Can you work these out from the drawing? Everything is in mm from the part's minimum corner. Give positions to 0.01 mm unless a question says otherwise; leave off trailing zeros. Write each loop counter-clockwise with the first axis right and the second up, starting at its lowest first coordinate (ties: lowest second). Pieces come first, ordered by that corner, then holes. Notation, with made-up numbers: M 11.5,15.25 L 19.5,15.25 A24 ccw 19.5,49.25 Z; hole C 36,25 d5. An arc over 180 degrees is marked long. One line per item, written item: value.
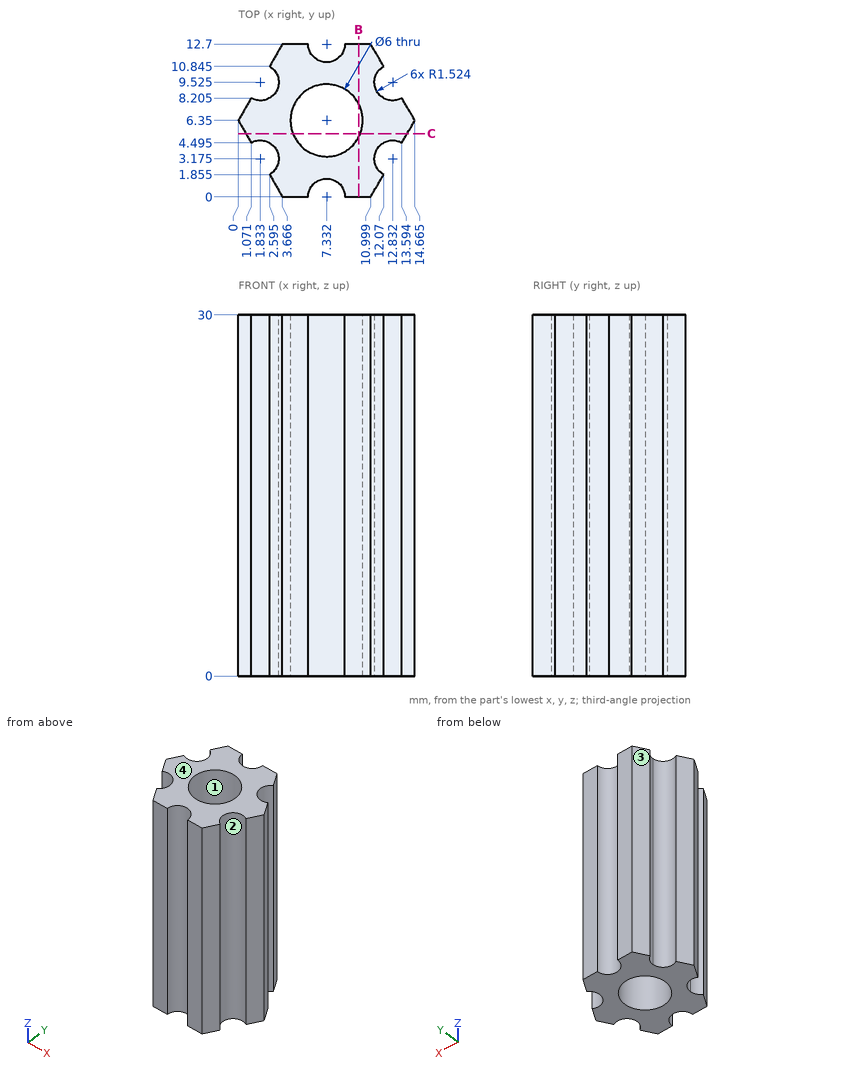
1) Please list where these lines run through material, in increasing order: L1, parallel to Y at x = 7.5, z = 19.75 (1 decimal); L2, parallel to Y at x = 5.5, z = 5.75 (1 decimal); L3, parallel to X at y = 8.5, z = 22.25 (1 decimal). Write a range as from..to.
Outcome:
L1: y = 1.5..3.4, 9.3..11.2
L2: y = 0..4, 8.7..12.7
L3: x = 3..5.2, 9.4..11.7
2) I'm going to push flat-ended pins straight in: pin 1 (1 mm diameter, centred on y = 11, z = 11, fed in from -X) (1 decimal); pin 2 (1 mm diameter, centred on y = 9, z = 9.5, fed in from -X). Where does each tip first touch, or does it pass through?
Outcome:
pin 1: stops at x = 2.6
pin 2: stops at x = 2.96
3) We'd pull the mould along Y, two halves only. Please class the marked faces 1, 2, 3 and 4: pulls with the +Y half, pulls with the -Y half, needs draft (parallel to the pull), parting line crosses it, or undercut.
Outcome:
face 1: undercut
face 2: undercut
face 3: pulls with the +Y half
face 4: needs draft
4) If we section it at C-C, the plane y = 5.25: Write out the boundary of the cut face in (x, z) (1 decimal).
Outcome:
outline: M 0.6,0 L 4.5,0 L 4.5,30 L 0.6,30 Z; M 10.1,0 L 14,0 L 14,30 L 10.1,30 Z
5) If we section it at B-B, the plane x = 10: Write out the boundary of the cut face in (y, z), then the cut area to 3 significant figures.
Outcome:
outline: M 0,0 L 4.98,0 L 4.98,30 L 0,30 Z; M 7.72,0 L 12.7,0 L 12.7,30 L 7.72,30 Z
area: 299 mm^2
